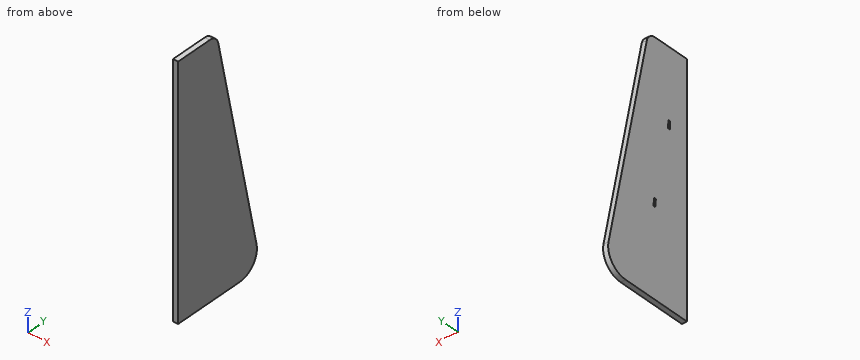
from build123d import *

# Parameters (mm, degrees)
BOSS_EXTRUDE1_DEPTH = 12.7
FILLET2_R           = 50.8
FILLET3_R           = 25.4
SKETCH2_W           = 20
SKETCH2_H           = 5
CUT_EXTRUDE1_DEPTH  = 5
SKETCH3_W           = 20
SKETCH3_H           = 5
CUT_EXTRUDE2_DEPTH  = 5


with BuildPart() as part:
    # Sketch1 → Boss-Extrude1 (new body)
    with BuildSketch(Plane(origin=(0, 0, 0), x_dir=(0, 0, -1), z_dir=(1, 0, 0))):
        Polygon((44.210163248, 18.673348758), (552.210163248, 18.673348758), (552.210163248, 259.973348758), (-61.277709779, 131.198589616), (-61.277709779, 18.673348758), align=None)
    extrude(amount=BOSS_EXTRUDE1_DEPTH)

    # Fillet2
    fillet2_edges = [part.edges().sort_by_distance(p)[0] for p in [
        (6.35, 259.973348758, -552.210163248),
    ]]
    fillet(fillet2_edges, radius=FILLET2_R)

    # Fillet3
    fillet3_edges = [part.edges().sort_by_distance(p)[0] for p in [
        (6.35, 131.198589616, 61.277709779),
    ]]
    fillet(fillet3_edges, radius=FILLET3_R)

    # Sketch2 → Cut-Extrude1 (cut)
    with BuildSketch(Plane(origin=(0, -2.351141299, -40.658116651), x_dir=(0, -0.05233595624294396, 0.998629534754574), z_dir=(-1, 0, 0))):
        with Locations((-83.722290221, 68.673348758)):
            Rectangle(SKETCH2_W, SKETCH2_H)
    extrude(amount=-CUT_EXTRUDE1_DEPTH, mode=Mode.SUBTRACT)

    # Sketch3 → Cut-Extrude2 (cut)
    with BuildSketch(Plane(origin=(0, -30.516141981, -7.826738697), x_dir=(0, -0.10452846326765375, 0.9945218953682733), z_dir=(-1, 0, 0))):
        with Locations((-330.716980881, 109.116306173)):
            Rectangle(SKETCH3_W, SKETCH3_H)
    extrude(amount=-CUT_EXTRUDE2_DEPTH, mode=Mode.SUBTRACT)


solid = part.part
CAD build for the part. Positions are in the model's coordinates, mm. Give positions to 0.01 mm unless a question says otherwise; leave off trailing zeros. Loops run counter-clockwise (first coordinate to the right, second up) from the corner with the lowest first, then second, coordinate; pieces in that order, holes last. Notation, with made-up numbers: M -5.5,88.5 L 45.5,88.5 A15 cw 45.5,97.5 Z; hole C 9,-24.5 d5. An arc over 180 degrees is marked long. Answer in a Markdown table with one row per item. Add a question column.
Item 1: Drop flat-ended pins along their axis: P1, Ø2, axis at x = 6.5, z = -44.5, coming from the +Y side; P2, Ø1.8, axis at y = 72, z = -120.5, coming from the -X side. Give the stop position or say it passes through.
Item 2: Band-saw the part on A-A on x = 2. Give the cut face in (y, z).
Item 3: Probe probe 1 along Y at (x, z) = (3, -323); probe 2 along Z at (x, y) = (9.25, 123.5); probe 3 along Y at (x, z) = (5.5, -128.5). List the from-to ranges inside material, lowest first.
Item 4: Band-saw the part on C-C on y = 162.5. Give the cut face in (x, z), then the cut area to 3 significant figures.
Item 5: Band-saw the part on B-B on z = -267. Give the cut face in (x, y).
Reply:
| question | item | result |
|---|---|---|
| 1 | P1 | stops at y = 153.61 |
| 1 | P2 | stops at x = 5 |
| 2 | outline | M 18.67,-552.21 L 197.4,-552.21 A50.8 ccw 247.12,-490.97 L 135.43,41.1 A25.4 ccw 110.58,61.28 L 18.67,61.28 Z; hole M 67.59,-110.82 L 68.64,-130.79 L 73.63,-130.53 L 72.58,-110.55 Z; hole M 109.04,-315.64 L 111.13,-335.53 L 116.1,-335.01 L 114.01,-315.12 Z |
| 3 | probe 1 | y = 18.67 to 109.81, 114.84 to 211.86 |
| 3 | probe 2 | z = -552.21 to 57.74 |
| 3 | probe 3 | y = 18.67 to 171.03 |
| 4 | outline | M 0,-552.21 L 12.7,-552.21 L 12.7,-87.84 L 0,-87.84 Z |
| 4 | area | 5,900 mm^2 |
| 5 | outline | M 0,18.67 L 12.7,18.67 L 12.7,200.11 L 0,200.11 Z |
